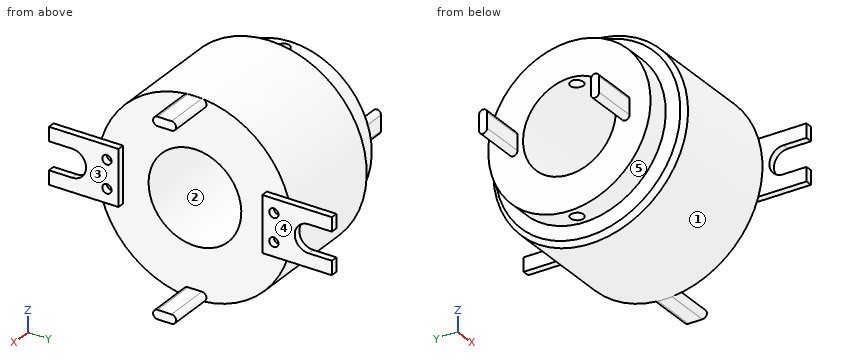
from build123d import *

# Parameters (mm, degrees)
SKETCH2_R           = 1.4
CUT_EXTRUDE1_DEPTH  = 10
CIRPATTERN1_COUNT   = 2
CHAMFER1_SIZE       = 1
BOSS_EXTRUDE1_DEPTH = 10
BOSS_EXTRUDE2_DEPTH = 10
SKETCH7_R           = 1
BOSS_EXTRUDE3_DEPTH = 1.5
CIRPATTERN2_COUNT   = 2


with BuildPart() as part:
    # Sketch1 → Revolve1 (revolve)
    with BuildSketch(Plane.XY, mode=Mode.PRIVATE) as revolve1_sk:
        Polygon((-13.027559055, 10), (18.472440945, 10), (18.472440945, 21), (-7.027559055, 21), (-7.027559055, 15.5), (-8.027559055, 15.5), (-8.027559055, 17.5), (-13.027559055, 17.5), align=None)
    revolve(revolve1_sk.sketch.rotate(Axis((-13.027559055, 0, 0), (1, 0, 0)), 90), axis=Axis((-13.027559055, 0, 0), (1, 0, 0)))

    # Sketch2 → Cut-Extrude1 (cut)
    with BuildSketch(Plane.XY.offset(17.5)):
        with Locations((-10.527559055, 0)):
            Circle(SKETCH2_R)
    cut_extrude1 = extrude(amount=-CUT_EXTRUDE1_DEPTH, mode=Mode.SUBTRACT)

    # CirPattern1: Cut-Extrude1 ×2 about axis
    cirpattern1_axis = Axis((-13.027559055, 0, 0), (-1, 0, 0))
    for i in range(1, CIRPATTERN1_COUNT):
        add(cut_extrude1.rotate(cirpattern1_axis, i * 360 / CIRPATTERN1_COUNT), mode=Mode.SUBTRACT)

    # Chamfer1
    chamfer1_edges = [part.edges().sort_by_distance(p)[0] for p in [
        (-7.027559055, 0, -21),
    ]]
    chamfer(chamfer1_edges, length=CHAMFER1_SIZE)

    # Sketch5 → Boss-Extrude1 (add)
    with BuildSketch(Plane.ZY.offset(13.027559055)):
        with BuildLine():
            Line((-1.622283046, 12.958236181), (1.622283046, 12.958236181))
            ThreePointArc((1.622283046, 12.958236181), (2.503523219, 12.076996008), (1.622283046, 11.195755835))
            Line((1.622283046, 11.195755835), (-1.622283046, 11.195755835))
            ThreePointArc((-1.622283046, 11.195755835), (-2.503523219, 12.076996008), (-1.622283046, 12.958236181))
        make_face()
        with BuildLine():
            Line((1.622283046, -12.958236181), (-1.622283046, -12.958236181))
            ThreePointArc((-1.622283046, -12.958236181), (-2.503523219, -12.076996008), (-1.622283046, -11.195755835))
            Line((-1.622283046, -11.195755835), (1.622283046, -11.195755835))
            ThreePointArc((1.622283046, -11.195755835), (2.503523219, -12.076996008), (1.622283046, -12.958236181))
        make_face()
    extrude(amount=BOSS_EXTRUDE1_DEPTH)

    # Sketch6 → Boss-Extrude2 (add)
    with BuildSketch(Plane(origin=(18.472440945, 0, 0), x_dir=(0, 0, -1), z_dir=(1, 0, 0))):
        with BuildLine():
            Line((-20.943347365, -1.505224441), (-20.943347365, 1.505224441))
            ThreePointArc((-20.943347365, 1.505224441), (-19.968101194, 2.480470612), (-18.992855023, 1.505224441))
            Line((-18.992855023, 1.505224441), (-18.992855023, -1.505224441))
            ThreePointArc((-18.992855023, -1.505224441), (-19.968101194, -2.480470612), (-20.943347365, -1.505224441))
        make_face()
        with BuildLine():
            Line((18.992855023, 1.505224441), (18.992855023, -1.505224441))
            ThreePointArc((18.992855023, -1.505224441), (19.968101194, -2.480470612), (20.943347365, -1.505224441))
            Line((20.943347365, -1.505224441), (20.943347365, 1.505224441))
            ThreePointArc((20.943347365, 1.505224441), (19.968101194, 2.480470612), (18.992855023, 1.505224441))
        make_face()
    extrude(amount=BOSS_EXTRUDE2_DEPTH)

    # Sketch7 → Boss-Extrude3 (add)
    with BuildSketch(Plane(origin=(18.472440945, 0, 0), x_dir=(0, 0, -1), z_dir=(1, 0, 0))):
        with BuildLine():
            Line((-6, 30.5), (-3, 30.5))
            Line((-3, 30.5), (-3, 25.5))
            ThreePointArc((-3, 25.5), (0, 22.5), (3, 25.5))
            Line((3, 25.5), (3, 30.5))
            Line((3, 30.5), (6, 30.5))
            Line((6, 30.5), (6, 15.5))
            Line((6, 15.5), (-6, 15.5))
            Line((-6, 15.5), (-6, 30.5))
        make_face()
        with Locations((-3, 18)):
            Circle(SKETCH7_R, mode=Mode.SUBTRACT)
        with Locations((3, 18)):
            Circle(SKETCH7_R, mode=Mode.SUBTRACT)
    boss_extrude3 = extrude(amount=BOSS_EXTRUDE3_DEPTH)

    # CirPattern2: Boss-Extrude3 ×2 about axis
    cirpattern2_axis = Axis((0, 0, 0), (1, 0, 0))
    for i in range(1, CIRPATTERN2_COUNT):
        add(boss_extrude3.rotate(cirpattern2_axis, i * 360 / CIRPATTERN2_COUNT))


solid = part.part
Can you work these out from the model? Positions are in its coordinate system, mm. Face numbers are marked on the shaded views. A direction names the side the tool comes from. Round coordinates to 2 decimals unless told otherwise and drop trailing zeros. Order: outer loops, then holes, each group sorted by start corner. A loop starts at its lowest first (then second) coordinate and runs counter-clockwise, first axis right, second up. Notation, with made-up numbers: (-37, 59) -> (-16, 59) arc R18 cw to (-16, 65) -> close; hole circle Ø3 at (84.5, -3). An arc over 180 degrees is marked (long way). Write each question's results on one line, items separated by ' | '. Start each with the question number.
Item 1: If we section it at B-B, the plane x = -18: Write out the boundary of the cut face in (y, z), then the cut area to 3 significant figures.
Item 2: Please list where these lines run through material, in increasing order: L1, parallel to Y at x = 0.5, z = -1.5; L2, parallel to Y at x = 12, z = 0; L3, parallel to X at y = 10.5, z = -13.5.
Item 3: Which directions (+Z, -Z, +X, -X, +Y, -Y) give clear straight access to the entire face, cutting with the end or side of a thin tool? Please do the marked faces 4 and 5.
Item 4: If we section it at D-D, the plane x = 8.5: Write out the boundary of the cut face in (y, z).
Item 5: Thinking about a two-plate mould opening in Y: for the marked faces 1, 2 and 3, which applies, +Y half, -Y half, draft (parallel to the pull), parting line (faces both ways), or undercut?
Item 6: Will these pins go through, and if not, where does the flat tip stop? pin 1 (3 mm diameter, centred on x = -10.53, y = 0, fed in from -Z); pin 2 (1.5 mm diameter, centred on y = 18.5, z = -11, fed in from -X); pin 3 (8 mm diameter, centred on x = -9, z = 14.5, fed in from -Y).
Results:
1) outline: (-12.96, -1.62) arc R0.88 ccw to (-11.2, -1.62) -> (-11.2, 1.62) arc R0.88 ccw to (-12.96, 1.62) -> close; (11.2, -1.62) arc R0.88 ccw to (12.96, -1.62) -> (12.96, 1.62) arc R0.88 ccw to (11.2, 1.62) -> close | area: 16.3 mm2
2) L1: y = -20.95 to -9.89, 9.89 to 20.95 | L2: y = -21 to -10, 10 to 21 | L3: x = -13.03 to -8.03, -7.03 to 18.47
3) face 4: +Z, -Z, +X, +Y, -Y | face 5: -X
4) outline: circle Ø42 at (0, 0); hole circle Ø20 at (0, 0)
5) face 1: parting line | face 2: undercut | face 3: draft
6) pin 1: stops at z = -17.5 | pin 2: stops at x = -6.25 | pin 3: stops at y = -17.36
